Geometry: final body of the model. Coordinates: model frame, mm. Face numbers are marked on the shaded views. Give positions to 0.01 mm unless a question says otherwise; leave off trailing zeros. Loops run counter-clockwise (first coordinate to the right, second up) from the corner with the lowest first, then second, coordinate; pieces in that order, holes last.
from build123d import *

# Parameters (mm, degrees)
PAD_DEPTH            = 155
SKETCH001_R          = 1.5
SKETCH001_W          = 13
SKETCH001_H          = 130
POCKET_DEPTH         = 12.001
SKETCH002_W          = 5.583172
SKETCH002_H          = 23.950112
POCKET001_DEPTH      = 25.001
POCKET001_DEPTH_BACK = -130.001
SKETCH003_W          = 22
SKETCH003_H          = 22
POCKET002_DEPTH      = 12.001
SKETCH004_W          = 11.5
SKETCH004_H          = 12.924639
POCKET003_DEPTH      = 31
SKETCH005_W          = 12
SKETCH005_H          = 25
PAD001_DEPTH         = 10
SKETCH006_R          = 1.35
POCKET004_DEPTH      = 155.001
SKETCH007_R          = 1.5
POCKET005_DEPTH      = 12.001003


with BuildPart() as part:
    # Sketch → Pad (new body)
    with BuildSketch(Plane.XY):
        with BuildLine():
            Line((39.5, 4.836187), (-20, 4.836187))
            Line((-20, 4.836187), (-20, -7.163813))
            ThreePointArc((20, -7.163813), (0, 0), (-20, -7.163813))
            Line((20, -7.163813), (39.5, -7.163813))
            Line((39.5, 4.836187), (39.5, -7.163813))
        make_face()
    extrude(amount=PAD_DEPTH)

    # Sketch001 → Pocket (cut, through all)
    with BuildSketch(Plane.XZ.offset(7.163813)):
        with Locations((28.5, 135)):
            Circle(SKETCH001_R)
        with Locations((34.5, 135)):
            Circle(SKETCH001_R)
        with Locations((33, 65)):
            Rectangle(SKETCH001_W, SKETCH001_H)
    extrude(amount=-POCKET_DEPTH, mode=Mode.SUBTRACT)

    # Sketch002 → Pocket001 (cut, two sides)
    with BuildSketch(Plane(origin=(0, 0, 130), x_dir=(1, 0, 0), z_dir=(0, 0, -1))) as pocket001_sk:
        with Locations((-19.791586, -0.240771)):
            Rectangle(SKETCH002_W, SKETCH002_H)
    extrude(amount=-POCKET001_DEPTH, mode=Mode.SUBTRACT)
    extrude(pocket001_sk.sketch, amount=-POCKET001_DEPTH_BACK, mode=Mode.SUBTRACT)

    # Sketch003 → Pocket002 (cut, through all)
    with BuildSketch(Plane(origin=(0, 4.836187, 0), x_dir=(-1, 0, 0), z_dir=(0, 1, 0))):
        with Locations((6, 41.7)):
            Rectangle(SKETCH003_W, SKETCH003_H)
    extrude(amount=-POCKET002_DEPTH, mode=Mode.SUBTRACT)

    # Sketch004 → Pocket003 (cut)
    with BuildSketch(Plane(origin=(0, 0, 0), x_dir=(1, 0, 0), z_dir=(0, 0, -1))):
        with Locations((-11.25, 0.936987)):
            Rectangle(SKETCH004_W, SKETCH004_H)
    extrude(amount=-POCKET003_DEPTH, mode=Mode.SUBTRACT)

    # Sketch005 → Pad001 (new body)
    with BuildSketch(Plane.YZ.offset(39.5)):
        with Locations((-1.16381, 142.5)):
            Rectangle(SKETCH005_W, SKETCH005_H)
    extrude(amount=PAD001_DEPTH)

    # Sketch006 → Pocket004 (cut, through all)
    with BuildSketch(Plane.XY.offset(155)):
        with Locations((39.5, -1.16381)):
            Circle(SKETCH006_R)
    extrude(amount=-POCKET004_DEPTH, mode=Mode.SUBTRACT)

    # Sketch007 → Pocket005 (cut, through all)
    with BuildSketch(Plane.XZ.offset(7.163813)):
        with Locations((27.5, 150)):
            Circle(SKETCH007_R)
        with Locations((33.5, 150)):
            Circle(SKETCH007_R)
        with Locations((45.5, 150)):
            Circle(SKETCH007_R)
        with Locations((45.5, 135)):
            Circle(SKETCH007_R)
    extrude(amount=-POCKET005_DEPTH, mode=Mode.SUBTRACT)


solid = part.part
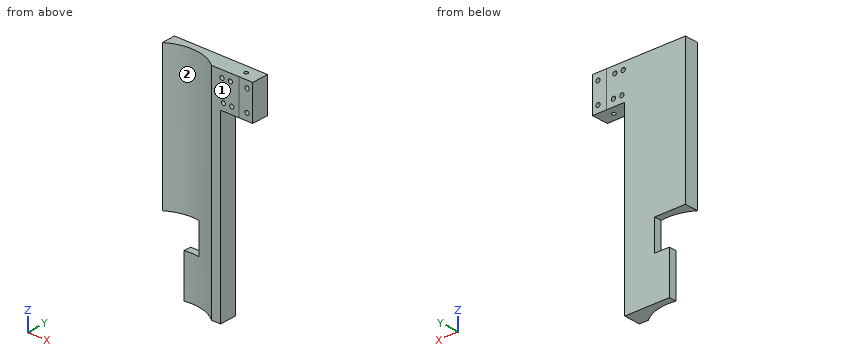
Item 1: Ray query, probe 1 along Z at (x, y) = (4, 0); probe 2 along Z at (x, y) = (33.5, 1.25); probe 3 along Z at (x, y) = (34.5, 0.5). Return the intervals inside material, ascending.
Values follow:
probe 1: z = 0 to 30.7, 52.7 to 155
probe 2: z = 130 to 133.88, 136.12 to 148.5, 151.5 to 155
probe 3: z = 130 to 133.5, 136.5 to 148.88, 151.12 to 155
Item 2: Pin query (flat end, axial travel): pin 1 (6 mm diameter, centred on y = -5.5, z = 103, fed in from -X); pin 2 (10 mm diameter, centred on x = 4.5, z = 118, fed in from -Y); pin 3 (2.5 mm diameter, centred on x = 45.5, z = 135, fed in from +Y); pin 4 (4.5 mm diameter, centred on x = 39.5, y = -1.16, fed in from -Z). Return the tip coordinate at first contact, or that it passes through.
Values follow:
pin 1: stops at x = -17
pin 2: stops at y = -1.47
pin 3: passes through
pin 4: stops at z = 130
Item 3: Draft query along X for the marked faces 1 and 2. Return one class per face: +X half, -X half, draft (parallel to the pull), parting line (faces both ways), or undercut.
Values follow:
face 1: draft
face 2: undercut
Item 4: Section query A-A on z = 135. Give the number of separate pieces and of enclosed holes in the cut face, plus the area to 3 significant figures.
Values follow:
separate pieces: 4
enclosed holes: 1
area: 492 mm2
Item 5: Section query C-C on z = 111.5. Return loops of the section in (x, y), plus the area to 3 significant figures.
Values follow:
outline: (-17, -4.98) arc R31.5 cw to (20, -7.16) - (26.5, -7.16) - (26.5, 4.84) - (-17, 4.84) - close
area: 330 mm2
Item 6: Section query B-B on z = 26.5. Return loops of the section in (x, y).
Values follow:
outline: (-5.5, -0.48) arc R31.5 cw to (20, -7.16) - (26.5, -7.16) - (26.5, 4.84) - (-5.5, 4.84) - close
